Source: CAD feature listing. Evaluate the final solid. Frame: model axes, mm. Give positions to 0.01 mm unless a question says otherwise; leave off trailing zeros. Order: outer loops, then holes, each group sorted by start corner. A loop starts at its lowest first (then second) coordinate and runs counter-clockwise, first axis right, second up.
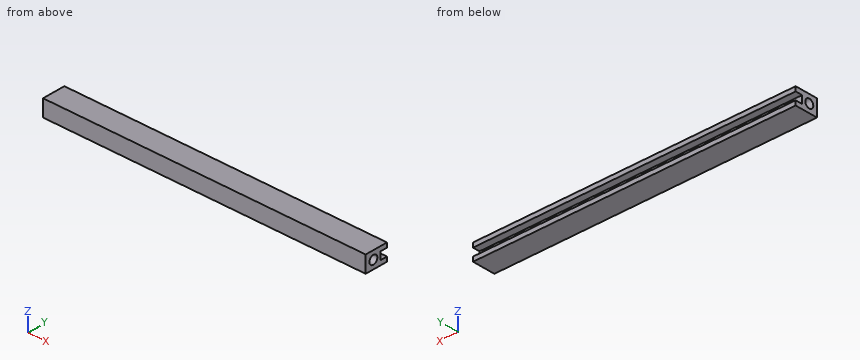
```python
from build123d import *

# Parameters (mm, degrees)
F1_DEPTH = 22.86
F2_W     = 320.04
F2_H     = 7.62
F3_DEPTH = 6.985
F4_R     = 4.269801
F5_DEPTH = 160.02


with BuildPart() as f1:
    # F0 (on Front) → F1 (new body)
    with BuildSketch(Plane.XZ):
        Polygon((160.02, 8.255), (-160.02, 8.255), (-160.02, 3.81), (-160.02, -3.81), (-160.02, -8.255), (160.02, -8.255), (160.02, -3.81), (160.02, 3.81), align=None)
    extrude(amount=F1_DEPTH)

    # F2 (on Front) → F3 (cut)
    with BuildSketch(Plane.XZ):
        Rectangle(F2_W, F2_H)
    extrude(amount=F3_DEPTH, mode=Mode.SUBTRACT)

    # F4 (on Right) → F5 (cut, symmetric)
    with BuildSketch(Plane.YZ):
        with Locations((-14.605, 0)):
            Circle(F4_R)
    extrude(amount=F5_DEPTH, both=True, mode=Mode.SUBTRACT)


solid = f1.part
```
1) Section query A-A, the plane y = -3. Return the cut outline in (x, z) (3 decimals).
Report:
outline: (-160.02, -8.255) - (160.02, -8.255) - (160.02, -3.81) - (-160.02, -3.81) - close; (-160.02, 3.81) - (160.02, 3.81) - (160.02, 8.255) - (-160.02, 8.255) - close
2) Pin query (flat end, axial travel): pin 1 (2.5 mm diameter, centred on x = -62.5, z = -0.5, fed in from +Y) (3 decimals). Return the tip coordinate at first contact, or that it passes through.
Report:
pin 1: stops at y = -6.985
3) Material intervals for L1, parallel to Y at x = -109.5, z = -0.25 (3 decimals); L2, parallel to Z at x = -81, y = -4.5 (3 decimals); L3, parallel to Y at x = 118.5, z = 0.5 (3 decimals), sorted ascending.
Report:
L1: y = -22.86 to -18.867, -10.343 to -6.985
L2: z = -8.255 to -3.81, 3.81 to 8.255
L3: y = -22.86 to -18.845, -10.365 to -6.985
4) Section query C-C, the plane x = -59. Return the cut outline in (y, z) (3 decimals).
Report:
outline: (-22.86, -8.255) - (0, -8.255) - (0, -3.81) - (-6.985, -3.81) - (-6.985, 3.81) - (0, 3.81) - (0, 8.255) - (-22.86, 8.255) - close; hole circle Ø8.54 at (-14.605, 0)
5) Section query B-B, the plane z = 0. Return the cut outline in (x, y) (3 decimals).
Report:
outline: (-160.02, -22.86) - (160.02, -22.86) - (160.02, -18.875) - (-160.02, -18.875) - close; (-160.02, -10.335) - (160.02, -10.335) - (160.02, -6.985) - (-160.02, -6.985) - close
